Check sheet for the modelled part. Datum: model origin and axes. Units: mm. A direction names the side the tool comes from. Round coordinates to 2 decimals unless told otherwise and drop trailing zeros. Write each loop counter-clockwise with the first axis right and the second up, starting at its lowest first coordinate (ties: lowest second). Pieces come first, ordered by that corner, then holes.
from build123d import *

# Parameters (mm, degrees)
SKETCH1_W           = 15
SKETCH1_H           = 10
BOSS_EXTRUDE1_DEPTH = 1
BOSS_EXTRUDE2_DEPTH = 1
BOSS_EXTRUDE3_DEPTH = 1
SKETCH4_W           = 4
SKETCH4_H           = 1
BOSS_EXTRUDE4_DEPTH = 0.05
LPATTERN1_COUNT     = 8
LPATTERN1_PITCH     = 1.2
FILLET1_R           = 0.5
BOSS_EXTRUDE5_DEPTH = 0.5
FILLET2_R           = 0.5


with BuildPart() as part:
    # Sketch1 → Boss-Extrude1 (new body)
    with BuildSketch(Plane(origin=(0, 0, 0), x_dir=(1, 0, 0), z_dir=(0, 1, 0))):
        Rectangle(SKETCH1_W, SKETCH1_H)
    extrude(amount=BOSS_EXTRUDE1_DEPTH)

    # Sketch2 → Boss-Extrude2 (add)
    with BuildSketch(Plane(origin=(0, 1, 0), x_dir=(1, 0, 0), z_dir=(0, 1, 0))):
        Polygon((7.5, -5), (7.5, -6), (2.5, -6), (1.5, -5), align=None)
    extrude(amount=-BOSS_EXTRUDE2_DEPTH)

    # Sketch3 → Boss-Extrude3 (add)
    with BuildSketch(Plane(origin=(0, 1, 0), x_dir=(1, 0, 0), z_dir=(0, 1, 0))):
        Polygon((0.5, -5), (0.5, -6), (-0.5, -6), (-1.5, -5), align=None)
    extrude(amount=-BOSS_EXTRUDE3_DEPTH)

    # Sketch4 → Boss-Extrude4 (add)
    with BuildSketch(Plane(origin=(0, 1, 0), x_dir=(1, 0, 0), z_dir=(0, 1, 0))):
        with Locations((-5.09817827, -4.25)):
            Rectangle(SKETCH4_W, SKETCH4_H)
    boss_extrude4 = extrude(amount=BOSS_EXTRUDE4_DEPTH)

    # LPattern1: Boss-Extrude4 ×8
    with Locations(*[(0, 0, -i * LPATTERN1_PITCH) for i in range(1, LPATTERN1_COUNT)]):
        add(boss_extrude4)

    # Fillet1
    fillet1_edges = [part.edges().sort_by_distance(p)[0] for p in [
        (-1.5, 0.5, 5),
        (1.5, 0.5, 5),
        (0.5, 0.5, 5),
        (2.5, 0.5, 6),
        (-0.5, 0.5, 6),
        (0.5, 0.5, 6),
        (7.5, 0.5, 6),
        (7.5, 0.5, -5),
        (-7.5, 0.5, -5),
        (-7.5, 0.5, 5),
    ]]
    fillet(fillet1_edges, radius=FILLET1_R - 0.0001)  # a hair under: the kernel refuses the full size

    # Sketch6 → Boss-Extrude5 (add)
    with BuildSketch(Plane.XZ):
        with BuildLine():
            Line((7.5, -5), (7.5, 6))
            Line((7.5, 6), (7, 6))
            ThreePointArc((7, 6), (6.073146166, 0.5), (7, -5))
            Line((7, -5), (7.5, -5))
        make_face()
    extrude(amount=BOSS_EXTRUDE5_DEPTH)

    # Fillet2
    fillet2_edges = [part.edges().sort_by_distance(p)[0] for p in [
        (7.5, -0.25, 6),
        (7.5, -0.25, -5),
    ]]
    fillet(fillet2_edges, radius=FILLET2_R - 0.0001)  # a hair under: the kernel refuses the full size


solid = part.part
1. Scan lines: line 1 along Z through (x, y) = (-4.75, 0.7); line 2 along X through (y, z) = (0.9, 5.25); line 3 along Y through (x, z) = (-4.25, -1.5). Record each from-to range of solid material in increasing order.
2. Go/stop test with a flat-tipped pin: pin 1 (1 mm diameter, centred on x = 4.5, z = 4, fed in from +Y). Record where the tip stops, or that it passes through.
3. Sectioned sample at B-B, the plane z = 0.5. Enter the section's corners in (x, y), plus the area to 3 significant figures.
4. Sectioned sample at D-D, the plane z = 3. Enter the section's corners in (x, y).
5. Sectioned sample at C-C, the plane x = 5. Enter the section's corners in (y, z), plus the area to 3 significant figures.
6. Set-up check for faces 1 (the cylindrical face through (6.073, -0.246, 0.578)), 2 (the flat face through (-5, 1.05, -3)), 3 (the flat face through (-4.4, 0.5, 5)): record each of +Z, -Z, +X, -X, +Y, -Y from which the full face is reachable in a straight line by a thin tool's end or side.
Computed values:
1. line 1: z = -5 to 5
1. line 2: x = -1.25 to 0.57, 1.75 to 7.5
1. line 3: y = 0 to 1.05
2. pin 1: stops at y = 1
3. outline: (-7.5, 0) - (6.07, 0) - (6.07, -0.5) - (7.5, -0.5) - (7.5, 1) - (-3.1, 1) - (-3.1, 1.05) - (-7.1, 1.05) - (-7.1, 1) - (-7.5, 1) - close
3. area: 15.9 mm2
4. outline: (-7.5, 0) - (6.26, 0) - (6.26, -0.5) - (7.5, -0.5) - (7.5, 1) - (-3.1, 1) - (-3.1, 1.05) - (-7.1, 1.05) - (-7.1, 1) - (-7.5, 1) - close
5. outline: (0, -5) - (1, -5) - (1, 6) - (0, 6) - close
5. area: 11.0 mm2
6. face 1: -X, -Y
6. face 2: +Z, -Z, +X, -X, +Y
6. face 3: +Z, -X, +Y, -Y
